Geometry: final body of the model. Coordinates: model frame, mm. Face numbers are marked on the shaded views. A direction names the side the tool comes from. Give positions to 0.01 mm unless a question says otherwise; leave off trailing zeros. Write each loop counter-clockwise with the first axis right and the second up, starting at its lowest first coordinate (ties: lowest second). Pieces come first, ordered by that corner, then holes. Notation, with made-up numbers: (45.25, 69) -> (76.25, 69) arc R20 ccw to (76.25, 101) -> close; hole circle Ø10 at (62, 82.5). An arc over 180 degrees is marked (long way). Answer as a JSON object with one key per item and string values.
from build123d import *

# Parameters (mm, degrees)
SKETCH1_R                  = 12.7
BOSS_EXTRUDE1_DEPTH        = 5.08
SKETCH2_R                  = 6.035
BOSS_EXTRUDE2_DEPTH        = 4.13
CUT_EXTRUDE1_REACH         = 22.184
SKETCH3_R                  = 3.1
CRVPATTERN1_OUTLINE_R      = 1.1303
CRVPATTERN1_DEPTH          = 5.08
SKETCH16_R                 = 2.05
CUT_EXTRUDE2_DEPTH         = 0.5
F_4_40_TAPPED_HOLE3_REACH  = 26.055
F_4_40_TAPPED_HOLE3_BORE_R = 1.1303
SKETCH24_R                 = 2.05
CUT_EXTRUDE3_DEPTH         = 7.1
F_4_40_TAPPED_HOLE4_REACH  = 26.104
F_4_40_TAPPED_HOLE4_BORE_R = 1.1303


# Read off the part's stored shape, not the designer's step: CrvPattern1
with BuildPart() as part:
    # Sketch1 → Boss-Extrude1 (new body)
    with BuildSketch(Plane.XY):
        Circle(SKETCH1_R)
    extrude(amount=BOSS_EXTRUDE1_DEPTH)

    # Sketch2 → Boss-Extrude2 (add)
    with BuildSketch(Plane.XY.offset(5.08)):
        Circle(SKETCH2_R)
    extrude(amount=BOSS_EXTRUDE2_DEPTH)

    # Sketch3 → Cut-Extrude1 (cut, up to next)
    with BuildSketch(Plane.XY.offset(9.21), mode=Mode.PRIVATE) as cut_extrude1_sk1:
        Circle(SKETCH3_R)
    cut_extrude1_tool1 = extrude(cut_extrude1_sk1.sketch, amount=-CUT_EXTRUDE1_REACH, mode=Mode.PRIVATE) & part.part
    add(cut_extrude1_tool1.solids().sort_by_distance((0, 0, 9.21))[0], mode=Mode.SUBTRACT)

    # Sketch10 → #4-40 Tapped Hole2 (revolve, cut)
    with BuildSketch(Plane(origin=(0.221066647, 9.527435622, 5.08), x_dir=(0, -1, 0), z_dir=(1, 0, 0))):
        Polygon((0, 0), (0, 8.279152758), (1.1303, 7.6), (1.1303, 0), align=None)
    revolve(axis=Axis((0.221066647, 9.527435622, 11.43), (0, 0, -1)), mode=Mode.SUBTRACT)

    # CrvPattern1 outline → CrvPattern1 (cut)
    with BuildSketch(Plane.XY):
        with Locations((-8.140467958, 4.955167144)):
            Circle(CRVPATTERN1_OUTLINE_R)
        with Locations((-8.361534605, -4.572268479)):
            Circle(CRVPATTERN1_OUTLINE_R)
        with Locations((-0.221066647, -9.527435622)):
            Circle(CRVPATTERN1_OUTLINE_R)
        with Locations((8.140467958, -4.955167144)):
            Circle(CRVPATTERN1_OUTLINE_R)
        with Locations((8.361534605, 4.572268479)):
            Circle(CRVPATTERN1_OUTLINE_R)
    extrude(amount=CRVPATTERN1_DEPTH, mode=Mode.SUBTRACT)

    # Sketch16 → Cut-Extrude2 (cut)
    with BuildSketch(Plane(origin=(6.035, 0, 9.21), x_dir=(0, 0, -1), z_dir=(1, 0, 0))):
        with Locations(Location((2.069027283, 0, 0), (0, 0, 90))):
            Circle(SKETCH16_R)
    extrude(amount=-CUT_EXTRUDE2_DEPTH, mode=Mode.SUBTRACT)

    # #4-40 Tapped Hole3 bore → #4-40 Tapped Hole3 (cut, up to next)
    with BuildSketch(Plane(origin=(5.535, 0, 0), x_dir=(0, 0, -1), z_dir=(1, 0, 0)), mode=Mode.PRIVATE) as f_4_40_tapped_hole3_sk1:
        with Locations((-7.140972717, 0)):
            Circle(F_4_40_TAPPED_HOLE3_BORE_R)
    f_4_40_tapped_hole3_tool1 = extrude(f_4_40_tapped_hole3_sk1.sketch, amount=-F_4_40_TAPPED_HOLE3_REACH, mode=Mode.PRIVATE) & part.part
    add(f_4_40_tapped_hole3_tool1.solids().sort_by_distance((5.535, 0, 7.140973))[0], mode=Mode.SUBTRACT)

    # Sketch24 → Cut-Extrude3 (cut)
    with BuildSketch(Plane(origin=(12.7, 0, 5.08), x_dir=(0, 0, -1), z_dir=(1, 0, 0))):
        with Locations(Location((2.585319139, 0, 0), (0, 0, 90))):
            Circle(SKETCH24_R)
    extrude(amount=-CUT_EXTRUDE3_DEPTH, mode=Mode.SUBTRACT)

    # #4-40 Tapped Hole4 bore → #4-40 Tapped Hole4 (cut, up to next)
    with BuildSketch(Plane(origin=(5.6, 0, 0), x_dir=(0, 0, -1), z_dir=(1, 0, 0)), mode=Mode.PRIVATE) as f_4_40_tapped_hole4_sk1:
        with Locations((-2.494680861, 0)):
            Circle(F_4_40_TAPPED_HOLE4_BORE_R)
    f_4_40_tapped_hole4_tool1 = extrude(f_4_40_tapped_hole4_sk1.sketch, amount=-F_4_40_TAPPED_HOLE4_REACH, mode=Mode.PRIVATE) & part.part
    add(f_4_40_tapped_hole4_tool1.solids().sort_by_distance((5.6, 0, 2.494681))[0], mode=Mode.SUBTRACT)


solid = part.part
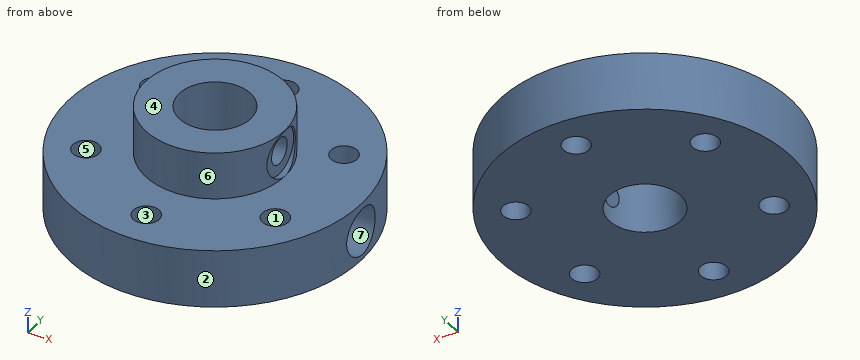
Q1. Cut plane D-D (z = 3). Return the cut outline in (x, y).
Values:
{"outline": "(2.93, -1.01) arc R3.1 cw (long way) to (2.93, 1.01) -> (5.6, 1.01) -> (5.6, 1.99) -> (12.54, 1.99) arc R12.7 ccw (long way) to (12.54, -1.99) -> (5.6, -1.99) -> (5.6, -1.01) -> close; hole circle Ø2.26 at (-8.36, -4.57); hole circle Ø2.26 at (-8.14, 4.96); hole circle Ø2.26 at (-0.22, -9.53); hole circle Ø2.26 at (0.22, 9.53); hole circle Ø2.26 at (8.14, -4.96); hole circle Ø2.26 at (8.36, 4.57)"}
Q2. Material intervals for L1, parallel to Y at x = -8, z = 4.5; L2, parallel to Y at x = 1.25, z = 4; L3, parallel to Y at x = -0.25, z = 2.5, sorted ascending. Write a range as from..to.
Values:
{"L1": "-9.86..-5.64, -3.5..3.83, 6.08..9.86", "L2": "-12.64..-2.84, 2.84..9.06, 10..12.64", "L3": "-12.7..-10.66, -8.4..-3.09, 3.09..8.5, 10.55..12.7"}
Q3. Cut plane C-C (z = 1). Return the cut outline in (x, y), and give its area (3 significant figures).
Values:
{"outline": "(5.6, -1.4) -> (5.6, 1.4) -> (12.62, 1.4) arc R12.7 ccw (long way) to (12.62, -1.4) -> close; hole circle Ø2.26 at (-8.36, -4.57); hole circle Ø2.26 at (-8.14, 4.96); hole circle Ø6.2 at (0, 0); hole circle Ø2.26 at (-0.22, -9.53); hole circle Ø2.26 at (0.22, 9.53); hole circle Ø2.26 at (8.14, -4.96); hole circle Ø2.26 at (8.36, 4.57)", "area": "433 mm²"}
Q4. Cut plane B-B (x = 7.75). Return the cut outline in (y, z), and give its area (3 significant figures).
Values:
{"outline": "(-10.06, 0) -> (-6.02, 0) -> (-6.02, 5.08) -> (-10.06, 5.08) -> close; (-3.89, 0) -> (3.62, 0) -> (3.62, 5.08) -> (-3.89, 5.08) -> close; (5.52, 0) -> (10.06, 0) -> (10.06, 5.08) -> (5.52, 5.08) -> close; hole circle Ø4.1 at (0, 2.49)", "area": "68.6 mm²"}
Q5. First-contact query: P1, Ø4, axis at y = 8.5, z = 3.5, coming from the -X side; P2, Ø2, axis at y = 2.5, z = 2, coming from the +X side; P3, Ø5, axis at y = 8.5, z = 2, coming from the +X side. Flat tips, straight axial feed; report the tip coordinate or a pass-through.
Values:
{"P1": "x = -10.91", "P2": "x = 12.58", "P3": "x = 11.19"}
Q6. Set-up query: the marked faces 5, 6 and 7. Return all of +Z, -Z, +X, -X, +Y, -Y with unobstructed straight access to the full face (end or side cutting, diameter ignored); none if empty.
Values:
{"face 5": "+Z, -Z", "face 6": "+Z", "face 7": "+X"}
Q7. Mould query, pull axis Y, two halves, no side actions, for the marked faces 1, 2, 3 and 4. Classes: pulls with the +Y half, pulls with the -Y half, needs draft (parallel to the pull), parting line crosses it, or undercut.
Values:
{"face 1": "undercut", "face 2": "parting line crosses it", "face 3": "undercut", "face 4": "needs draft"}
Q8. Cut plane A-A (y = 0). Return the cut outline in (x, z) (3 decimals), and give its area (3 significant figures).
Values:
{"outline": "(-12.7, 0) -> (-3.1, 0) -> (-3.1, 9.21) -> (-6.035, 9.21) -> (-6.035, 5.08) -> (-12.7, 5.08) -> close; (3.1, 0) -> (12.7, 0) -> (12.7, 0.445) -> (5.6, 0.445) -> (5.6, 1.364) -> (3.1, 1.364) -> close; (3.1, 3.625) -> (5.6, 3.625) -> (5.6, 4.545) -> (12.7, 4.545) -> (12.7, 5.08) -> (6.035, 5.08) -> (6.035, 5.091) -> (5.535, 5.091) -> (5.535, 6.011) -> (3.1, 6.011) -> close; (3.1, 8.271) -> (5.535, 8.271) -> (5.535, 9.191) -> (6.035, 9.191) -> (6.035, 9.21) -> (3.1, 9.21) -> close", "area": "79.5 mm²"}
